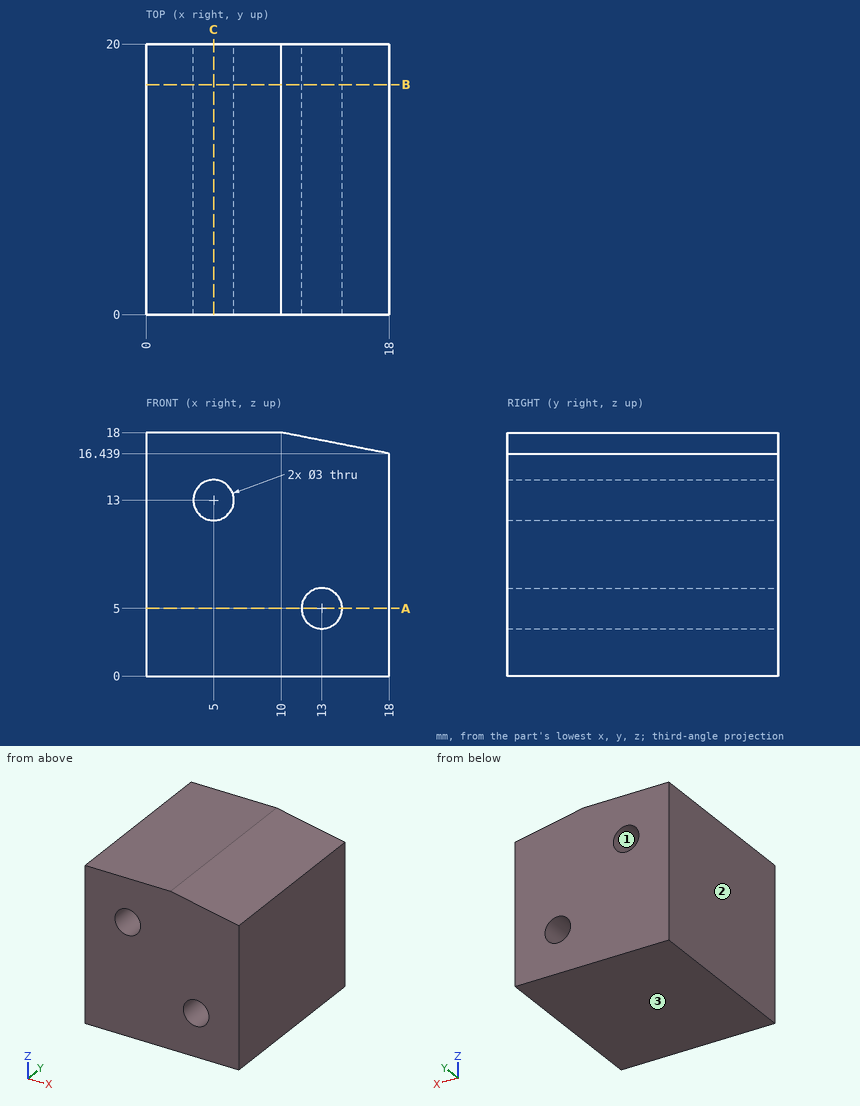
Geometry: see drawing. Coordinates: mm, zero at the bounding-box minimum. Give positions to 0.01 mm unless a question says otherwise; leave off trailing zeros. Loops run counter-clockwise (first coordinate to the right, second up) from the corner with the lowest first, then second, coordinate; pieces in that order, holes last. Notation, with made-up numbers: (46.25, -38.75) - (98.25, -38.75) arc R28 ccw to (98.25, -16.75) - close; hole circle Ø2 at (58, 48). An arc over 180 degrees is marked (long way). One line per question, with ' | ' between items. Start each with the question number.
(1) Section query B-B on y = 17. Return loops of the section in (x, z), then the cut area to 3 significant figures.
(2) Section query A-A on z = 5. Return loops of the section in (x, y).
(3) Pull-direction query (X, two-part tool) for the marked faces 1, 2 and 3; classes: released by +X, released by -X, zero draft, split by the parting line, or undercut.
(4) Section query C-C on x = 5. Return loops of the section in (y, z), then the cut area to 3 significant figures.
(5) Contact query for flat-ended pins moving along their axis: pin 1 (6 mm diameter, centred on x = 11.5, z = 3, fed in from -Y); pin 2 (2.5 mm diameter, centred on x = 13, z = 5, fed in from -Y); pin 3 (2 mm diameter, centred on x = 12, y = 5, fed in from +Z). Output: stop coordinate, or through.
(6) Ray query, line 1 (Z direction, x = 5, y = 6.25); line 2 (X direction, y = 2.5, z = 4.5); line 3 (Z direction, x = 13, y = 10.75). Return the intervals inside material, ascending. Write a range as from..to.
The answers:
1) outline: (0, 0) - (18, 0) - (18, 16.44) - (10, 18) - (0, 18) - close; hole circle Ø3 at (5, 13); hole circle Ø3 at (13, 5) | area: 304 mm2
2) outline: (0, 0) - (11.5, 0) - (11.5, 20) - (0, 20) - close; (14.5, 0) - (18, 0) - (18, 20) - (14.5, 20) - close
3) face 1: undercut | face 2: released by -X | face 3: zero draft
4) outline: (0, 0) - (20, 0) - (20, 11.5) - (0, 11.5) - close; (0, 14.5) - (20, 14.5) - (20, 18) - (0, 18) - close | area: 300 mm2
5) pin 1: y = 0 | pin 2: through | pin 3: z = 17.8
6) line 1: 0..11.5, 14.5..18 | line 2: 0..11.59, 14.41..18 | line 3: 0..3.5, 6.5..17.41
